```python
from build123d import *

# Parameters (mm, degrees)
CROQUIS1_R              = 5
SALIENTE_EXTRUIR1_DEPTH = 250


with BuildPart() as part:
    # Croquis1 → Saliente-Extruir1 (new body)
    with BuildSketch(Plane(origin=(0, 0, 0), x_dir=(1, 0, 0), z_dir=(0, 1, 0))):
        with Locations(Location((0, 0, 0), (0, 0, 270))):
            Circle(CROQUIS1_R)
    extrude(amount=SALIENTE_EXTRUIR1_DEPTH)

    # Saliente-Extruir2 cone 1 section (on through the dimple's axis) → Saliente-Extruir2 (revolve)
    with BuildSketch(Plane(origin=(0, 250, 0), x_dir=(0, 0, -1), z_dir=(1, 0, 0))):
        Polygon((0, 0), (5, 0), (0, 5), align=None)
    revolve(axis=Axis((0, 250, 0), (0, 1, 0)))

    # Saliente-Extruir3 cone 1 section (on through the dimple's axis) → Saliente-Extruir3 (revolve)
    with BuildSketch(Plane(origin=(0, 0, 0), x_dir=(0, 0, 1), z_dir=(1, 0, 0))):
        Polygon((0, 0), (5, 0), (0, 5), align=None)
    revolve(axis=Axis((0, 0, 0), (0, -1, 0)))


solid = part.part
```
Here's how the part is built. I have some questions about the finished solid (model axes, mm). Round coordinates to 2 decimals unless told otherwise and drop trailing zeros. Loops run counter-clockwise (first coordinate to the right, second up) from the corner with the lowest first, then second, coordinate; pieces in that order, holes last. Notation, with made-up numbers: (-7, 61.5) -> (32, 61.5) arc R20 cw to (32, 83.5) -> close; hole circle Ø1 at (47.5, 86). An arc over 180 degrees is marked (long way). Answer as CSV lines item,"result". Start each with the question number.
1. I'm going to push flat-ended pins straight in: P1, Ø2, axis at x = -3.5, z = 0, coming from the +Y side; P2, Ø1, axis at y = 114.5, z = 1.5, coming from the +X side; P3, Ø5, axis at x = 3, z = 3, coming from the +Y side. Where does each tip first touch, or does it pass through?
2. I need wall thicknesses on probe 1 along X at (y, z) = (207, -0.25); probe 2 along X at (y, z) = (71.5, -3.5); probe 3 along Z at (x, y) = (4, 24). Which ranges of each line are inside material? Lowest first, please. Write a range as from..to.
3. Imagine slicing it at A-A on y = 216. Write out the boundary of the cut face in (x, z).
Solution:
1,P1,"y = 252.5"
1,P2,"x = 4.9"
1,P3,"y = 253.26"
2,probe 1,"-4.99..4.99"
2,probe 2,"-3.57..3.57"
2,probe 3,"-3..3"
3,outline,"circle Ø10 at (0, 0)"
